from build123d import *

# Parameters (mm, degrees)
SKETCH1_R                        = 5.3578125
BOSS_EXTRUDE1_DEPTH              = 6.35
FILLET1_R                        = 6.35
F_17_64_0_26563_DIAMETER_HOLE1_D = 6.747002


with BuildPart() as part:
    # Sketch1 → Boss-Extrude1 (new body)
    with BuildSketch(Plane.XY):
        Polygon((128.546632935, 292.971606529), (382.546632935, 292.971606529), (776.246632935, -872.634633965), (-265.153367065, -872.634633965), align=None)
        with Locations((396.756156044, 191.371606529)):
            Circle(SKETCH1_R, mode=Mode.SUBTRACT)
        with Locations((114.659199441, 192.325199783)):
            Circle(SKETCH1_R, mode=Mode.SUBTRACT)
        with Locations((-193.570796303, -720.234633965)):
            Circle(SKETCH1_R, mode=Mode.SUBTRACT)
        with Locations((704.664062174, -720.234633965)):
            Circle(SKETCH1_R, mode=Mode.SUBTRACT)
        with Locations((491.127459301, -88.028393471)):
            Circle(SKETCH1_R, mode=Mode.SUBTRACT)
        with Locations((593.220051006, -390.288393471)):
            Circle(SKETCH1_R, mode=Mode.SUBTRACT)
        with Locations((19.96580657, -88.028393471)):
            Circle(SKETCH1_R, mode=Mode.SUBTRACT)
        with Locations((-82.126785136, -390.288393471)):
            Circle(SKETCH1_R, mode=Mode.SUBTRACT)
        with Locations((306.346632935, 271.727158802)):
            Circle(SKETCH1_R, mode=Mode.SUBTRACT)
        with Locations((204.746632935, 271.727158802)):
            Circle(SKETCH1_R, mode=Mode.SUBTRACT)
        with Locations((-82.126785136, -834.534633965)):
            Circle(SKETCH1_R, mode=Mode.SUBTRACT)
        with Locations((593.220051006, -834.534633965)):
            Circle(SKETCH1_R, mode=Mode.SUBTRACT)
        with BuildLine():
            Line((-180.239726648, -736.327985402), (-172.111642745, -712.26360816))
            ThreePointArc((-172.111642745, -712.26360816), (-156.015412172, -704.29546149), (-148.047265502, -720.391692063))
            Line((-148.047265502, -720.391692063), (-156.175349405, -744.456069305))
            ThreePointArc((-156.175349405, -744.456069305), (-172.271579978, -752.424215975), (-180.239726648, -736.327985402))
        make_face(mode=Mode.SUBTRACT)
        with BuildLine():
            Line((-94.231734473, -791.354633965), (-68.831734473, -791.354633965))
            ThreePointArc((-68.831734473, -791.354633965), (-56.131734473, -804.054633965), (-68.831734473, -816.754633965))
            Line((-68.831734473, -816.754633965), (-94.231734473, -816.754633965))
            ThreePointArc((-94.231734473, -816.754633965), (-106.931734473, -804.054633965), (-94.231734473, -791.354633965))
        make_face(mode=Mode.SUBTRACT)
        with BuildLine():
            Line((580.520051006, -791.354633965), (605.920051006, -791.354633965))
            ThreePointArc((605.920051006, -791.354633965), (618.620051006, -804.054633965), (605.920051006, -816.754633965))
            Line((605.920051006, -816.754633965), (580.520051006, -816.754633965))
            ThreePointArc((580.520051006, -816.754633965), (567.820051006, -804.054633965), (580.520051006, -791.354633965))
        make_face(mode=Mode.SUBTRACT)
        with BuildLine():
            Line((-68.772097635, -406.311820835), (-60.644013732, -382.247443592))
            ThreePointArc((-60.644013732, -382.247443592), (-44.54778316, -374.279296923), (-36.57963649, -390.375527495))
            Line((-36.57963649, -390.375527495), (-44.707720392, -414.439904738))
            ThreePointArc((-44.707720392, -414.439904738), (-60.803950965, -422.408051408), (-68.772097635, -406.311820835))
        make_face(mode=Mode.SUBTRACT)
        with BuildLine():
            Line((33.202373314, -104.401534553), (41.330457217, -80.33715731))
            ThreePointArc((41.330457217, -80.33715731), (57.426687789, -72.36901064), (65.394834459, -88.465241213))
            Line((65.394834459, -88.465241213), (57.266750557, -112.529618456))
            ThreePointArc((57.266750557, -112.529618456), (41.170519984, -120.497765125), (33.202373314, -104.401534553))
        make_face(mode=Mode.SUBTRACT)
        with BuildLine():
            Line((127.949253412, 176.110415433), (136.077337315, 200.174792676))
            ThreePointArc((136.077337315, 200.174792676), (152.173567887, 208.142939345), (160.141714557, 192.046708773))
            Line((160.141714557, 192.046708773), (152.013630654, 167.98233153))
            ThreePointArc((152.013630654, 167.98233153), (135.917400082, 160.01418486), (127.949253412, 176.110415433))
        make_face(mode=Mode.SUBTRACT)
        with BuildLine():
            Line((192.113515822, 253.947158802), (217.513515822, 253.947158802))
            ThreePointArc((217.513515822, 253.947158802), (230.213515822, 241.247158802), (217.513515822, 228.547158802))
            Line((217.513515822, 228.547158802), (192.113515822, 228.547158802))
            ThreePointArc((192.113515822, 228.547158802), (179.413515822, 241.247158802), (192.113515822, 253.947158802))
        make_face(mode=Mode.SUBTRACT)
        with BuildLine():
            Line((293.646632935, 253.947158802), (319.046632935, 253.947158802))
            ThreePointArc((319.046632935, 253.947158802), (331.746632935, 241.247158802), (319.046632935, 228.547158802))
            Line((319.046632935, 228.547158802), (293.646632935, 228.547158802))
            ThreePointArc((293.646632935, 228.547158802), (280.946632935, 241.247158802), (293.646632935, 253.947158802))
        make_face(mode=Mode.SUBTRACT)
        with BuildLine():
            Line((359.065010443, 168.025630302), (350.936926541, 192.090007545))
            ThreePointArc((350.936926541, 192.090007545), (358.905073211, 208.186238118), (375.001303783, 200.218091448))
            Line((375.001303783, 200.218091448), (383.129387686, 176.153714205))
            ThreePointArc((383.129387686, 176.153714205), (375.161241016, 160.057483633), (359.065010443, 168.025630302))
        make_face(mode=Mode.SUBTRACT)
        with BuildLine():
            Line((453.826515314, -112.529618456), (445.698431411, -88.465241213))
            ThreePointArc((445.698431411, -88.465241213), (453.666578081, -72.36901064), (469.762808654, -80.33715731))
            Line((469.762808654, -80.33715731), (477.890892557, -104.401534553))
            ThreePointArc((477.890892557, -104.401534553), (469.922745887, -120.497765125), (453.826515314, -112.529618456))
        make_face(mode=Mode.SUBTRACT)
        with BuildLine():
            Line((555.800986263, -414.439904738), (547.67290236, -390.375527495))
            ThreePointArc((547.67290236, -390.375527495), (555.64104903, -374.279296923), (571.737279603, -382.247443592))
            Line((571.737279603, -382.247443592), (579.865363506, -406.311820835))
            ThreePointArc((579.865363506, -406.311820835), (571.897216836, -422.408051408), (555.800986263, -414.439904738))
        make_face(mode=Mode.SUBTRACT)
        with BuildLine():
            Line((667.268615276, -744.456069305), (659.140531373, -720.391692063))
            ThreePointArc((659.140531373, -720.391692063), (667.108678043, -704.29546149), (683.204908616, -712.26360816))
            Line((683.204908616, -712.26360816), (691.332992518, -736.327985402))
            ThreePointArc((691.332992518, -736.327985402), (683.364845848, -752.424215975), (667.268615276, -744.456069305))
        make_face(mode=Mode.SUBTRACT)
    extrude(amount=BOSS_EXTRUDE1_DEPTH)

    # Fillet1
    fillet1_edges = [part.edges().sort_by_distance(p)[0] for p in [
        (128.546632935, 292.971606529, 3.175),
        (382.546632935, 292.971606529, 3.175),
        (776.246632935, -872.634633965, 3.175),
        (-265.153367065, -872.634633965, 3.175),
    ]]
    fillet(fillet1_edges, radius=FILLET1_R)

    # 17/64 (0.26563) Diameter Hole1 (through all)
    with Locations(Plane.XY.offset(6.35)):
        with Locations((-23.853367065, -269.384633965), (534.946632935, -269.384633965), (592.096632935, -777.384633965), (-81.003367065, -777.384633965)):
            Hole(F_17_64_0_26563_DIAMETER_HOLE1_D / 2)


solid = part.part
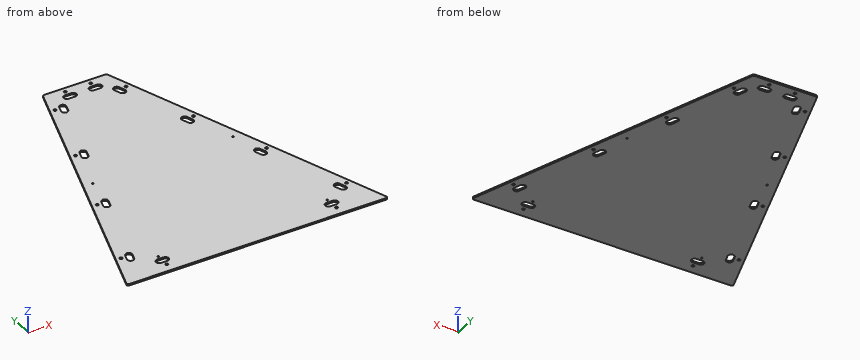
Could you check a few things on this model? Use its own coordinates, in mm. Give positions to 0.01 mm unless a question says otherwise; leave off trailing zeros. Order: outer loops, then holes, each group sorted by start corner. A loop starts at its lowest first (then second) coordinate and runs counter-clockwise, first axis right, second up.
Item 1: I'm going to push flat-ended pins straight in: pin 1 (1.5 mm diameter, centred on y = 9.5, z = 1.5, fed in from +X); pin 2 (1 mm diameter, centred on y = -390, z = 4, fed in from -X); pin 3 (3 mm diameter, centred on y = -113, z = 5, fed in from -X). Where does each tip first touch, or does it pass through?
Item 2: If we section it at C-C, the plane x = 513.5: Write out the boundary of the cut face in (y, z), plus the area to 3 significant figures.
Item 3: If we section it at A-A, the plane z = 5: Count the separate pieces of the cut face and the enclosed holes in it, plus the area to 3 significant figures.
Item 4: I need wall thicknesses on line 1 (X direction, y = 181.5, z = 1); line 2 (X direction, y = -747.5, z = 5); line 3 (Y direction, x = 326, z = 2.5). Which ranges of each line are inside material? Lowest first, please.
Item 5: If we section it at B-B, the plane y = -445.5: Write out the boundary of the cut face in (x, z).
Values:
1. pin 1: stops at x = 478.55
1. pin 2: stops at x = -102.31
1. pin 3: stops at x = -9.08
2. outline: (-872.63, 0) - (-94.73, 0) - (-94.73, 6.35) - (-872.63, 6.35) - close
2. area: 4,940 mm2
3. separate pieces: 1
3. enclosed holes: 28
3. area: 740,000 mm2
4. line 1: x = 90.9 to 129.77, 156.58 to 354.51, 381.32 to 420.2
4. line 2: x = -222.89 to -178.73, -157.68 to 668.78, 689.83 to 733.98
4. line 3: y = -872.63 to 230.62, 251.87 to 292.97
5. outline: (-120.88, 0) - (631.98, 0) - (631.98, 6.35) - (-120.88, 6.35) - close
